Print and shaded views of the part. All mm, measured from the part's lowest x, y and z. Round coordinates to 2 decimals unless told otherwise and drop trailing zeros. Order: outer loops, then holes, each group sorted by start corner. A loop starts at its lowest first (then second) coordinate and runs counter-clockwise, first axis right, second up. Notation, with made-up numbers: M -28.5,66 L -0.5,66 A31 ccw -0.5,95 Z; hole C 56,68 d2. An arc over 180 degrees is marked long. Write each question's results on one line, items separated by ' | '. Start each with the question number.
1. Drop a flat-ended pin along its axis: pin 1 Ø3 at (x, z) = (37, 15.5) entering from +Y. Give the stop position or say it passes through.
2. Band-saw the part on A-A, the plane z = 15. List the corners of the cut face in (x, y), then the cut area to 3 significant figures.
3. Band-saw the part on B-B, the plane x = 30. List the corners of the cut face in (y, z).
4. Band-saw the part on C-C, the plane y = 4. List the corners of the cut face in (x, z).
5. Two-plate mould, pull along Y, no slides. Class the marked faces 1 and 2: +Y half, -Y half, draft (parallel to the pull), parting line (faces both ways), or undercut.
6. Probe L1, parallel to X at y = 3.75, z = 15; L2, parallel to X at y = 10.6, z = 15; L3, parallel to Y at x = 31.5, z = 21.5. List the from-to ranges inside material, lowest first. Write a range as [from, to].
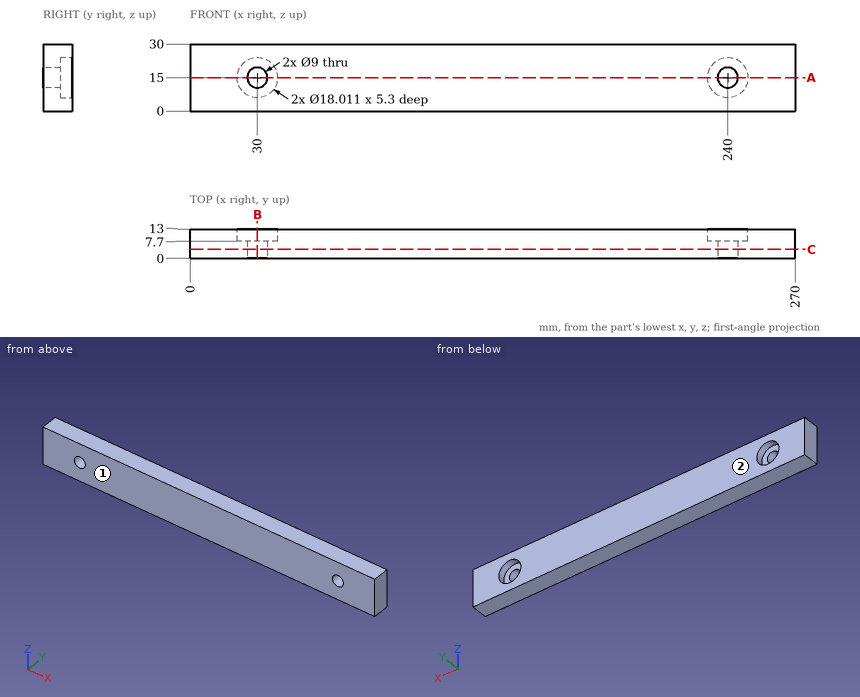
Solution:
1) pin 1: y = 7.7
2) outline: M 0,0 L 25.5,0 L 25.5,7.7 L 20.99,7.7 L 20.99,13 L 0,13 Z; M 34.5,0 L 235.5,0 L 235.5,7.7 L 230.99,7.7 L 230.99,13 L 39.01,13 L 39.01,7.7 L 34.5,7.7 Z; M 244.5,0 L 270,0 L 270,13 L 249.01,13 L 249.01,7.7 L 244.5,7.7 Z | area: 3,180 mm^2
3) outline: M 0,0 L 13,0 L 13,5.99 L 7.7,5.99 L 7.7,10.5 L 0,10.5 Z; M 0,19.5 L 7.7,19.5 L 7.7,24.01 L 13,24.01 L 13,30 L 0,30 Z
4) outline: M 0,0 L 270,0 L 270,30 L 0,30 Z; hole C 30,15 d9; hole C 240,15 d9
5) face 1: -Y half | face 2: +Y half
6) L1: [0, 25.5], [34.5, 235.5], [244.5, 270] | L2: [0, 20.99], [39.01, 230.99], [249.01, 270] | L3: [0, 7.7]
